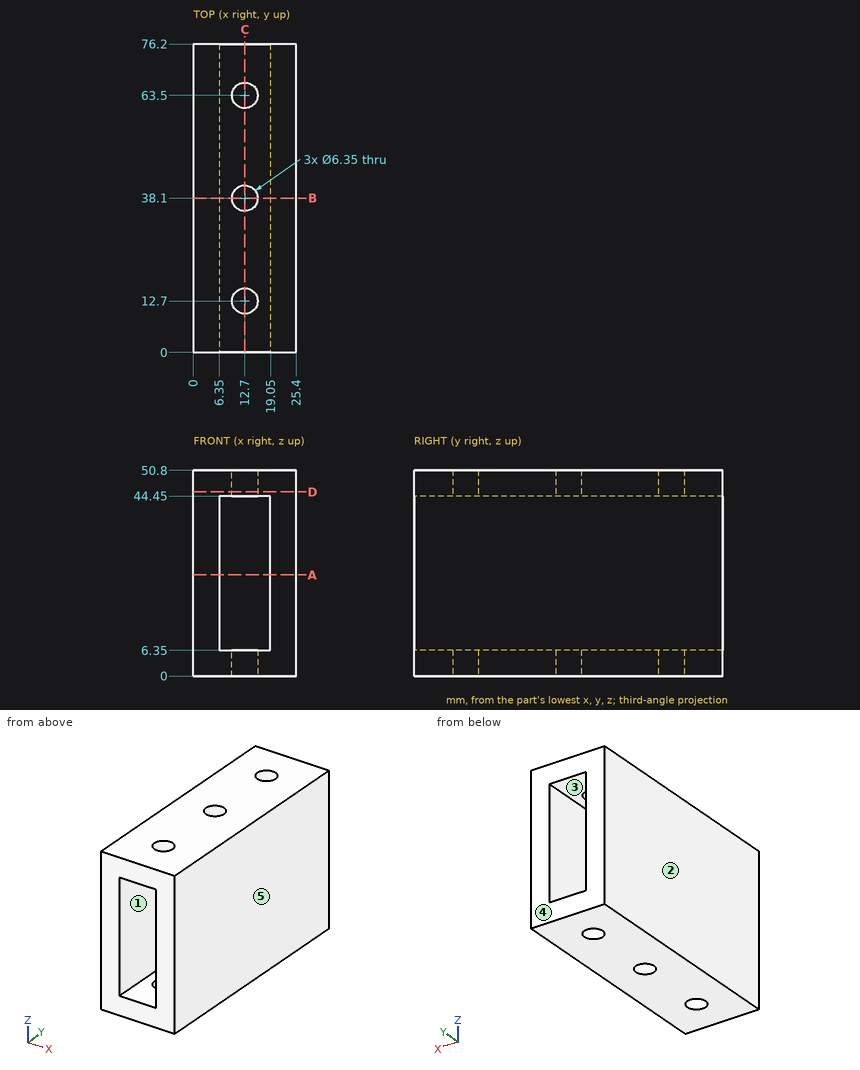
Print and shaded views of the part. All mm, measured from the part's lowest x, y and z. A direction names the side the tool comes from. Give positions to 0.01 mm unless a question says otherwise; leave off trailing zeros. Write each loop counter-clockwise with the first axis right and the second up, starting at its lowest first coordinate (ties: lowest second). Pieces come first, ordered by that corner, then holes. Notation, with made-up numbers: (26, 86) - (65, 86) arc R21 ccw to (65, 118) - close; hole circle Ø8 at (14.5, 1.5). An arc over 180 degrees is marked (long way). One line per question, with ' | ' between items. Start each with the question number.
(1) Slice it at C-C on x = 12.7. Give the number of separate pieces and of enclosed holes in the cut face, plus the area to 3 significant figures.
(2) Slice it at A-A on z = 25. Write the cut outline in (x, y), plus the area to 3 significant figures.
(3) Slice it at D-D on z = 45.5. Write the cut outline in (x, y) (3 decimals).
(4) Wall check: line 1 along Y through (x, z) = (12.7, 1.5) (3 decimals); line 2 along X through (y, z) = (52, 14); line 3 along Z through (x, y) = (15.5, 5). Give the ranges that are in metal, low to high. Write a range as from..to.
(5) Two-plate mould, pull along X, no slides. Class the marked faces 3, 4 and 5: +X half, -X half, draft (parallel to the pull), parting line (faces both ways), or undercut.
(6) 3-axis set-ups, long thin cutter, end or side, ignore diameter. For the marked faces 1 and 2: which of +Z, -Z, +X, -X, +Y, -Y reach the whole face in a straight line?
(7) Pin check, flat tip, straight feed: P1, Ø5.5, axis at x = 12.7, y = 38.1, coming from the +Z side. Stop position of the tip, or through.
(8) Slice it at B-B on y = 38.1. Write the cut outline in (x, z) (3 decimals).
Results below:
1) separate pieces: 8 | enclosed holes: 0 | area: 726 mm^2
2) outline: (0, 0) - (6.35, 0) - (6.35, 76.2) - (0, 76.2) - close; (19.05, 0) - (25.4, 0) - (25.4, 76.2) - (19.05, 76.2) - close | area: 968 mm^2
3) outline: (0, 0) - (25.4, 0) - (25.4, 76.2) - (0, 76.2) - close; hole circle Ø6.35 at (12.7, 12.7); hole circle Ø6.35 at (12.7, 38.1); hole circle Ø6.35 at (12.7, 63.5)
4) line 1: 0..9.525, 15.875..34.925, 41.275..60.325, 66.675..76.2 | line 2: 0..6.35, 19.05..25.4 | line 3: 0..6.35, 44.45..50.8
5) face 3: undercut | face 4: draft | face 5: +X half
6) face 1: +Y, -Y | face 2: +Z, -Z, -X, +Y, -Y
7) P1: through
8) outline: (0, 0) - (9.525, 0) - (9.525, 6.35) - (6.35, 6.35) - (6.35, 44.45) - (9.525, 44.45) - (9.525, 50.8) - (0, 50.8) - close; (15.875, 0) - (25.4, 0) - (25.4, 50.8) - (15.875, 50.8) - (15.875, 44.45) - (19.05, 44.45) - (19.05, 6.35) - (15.875, 6.35) - close
